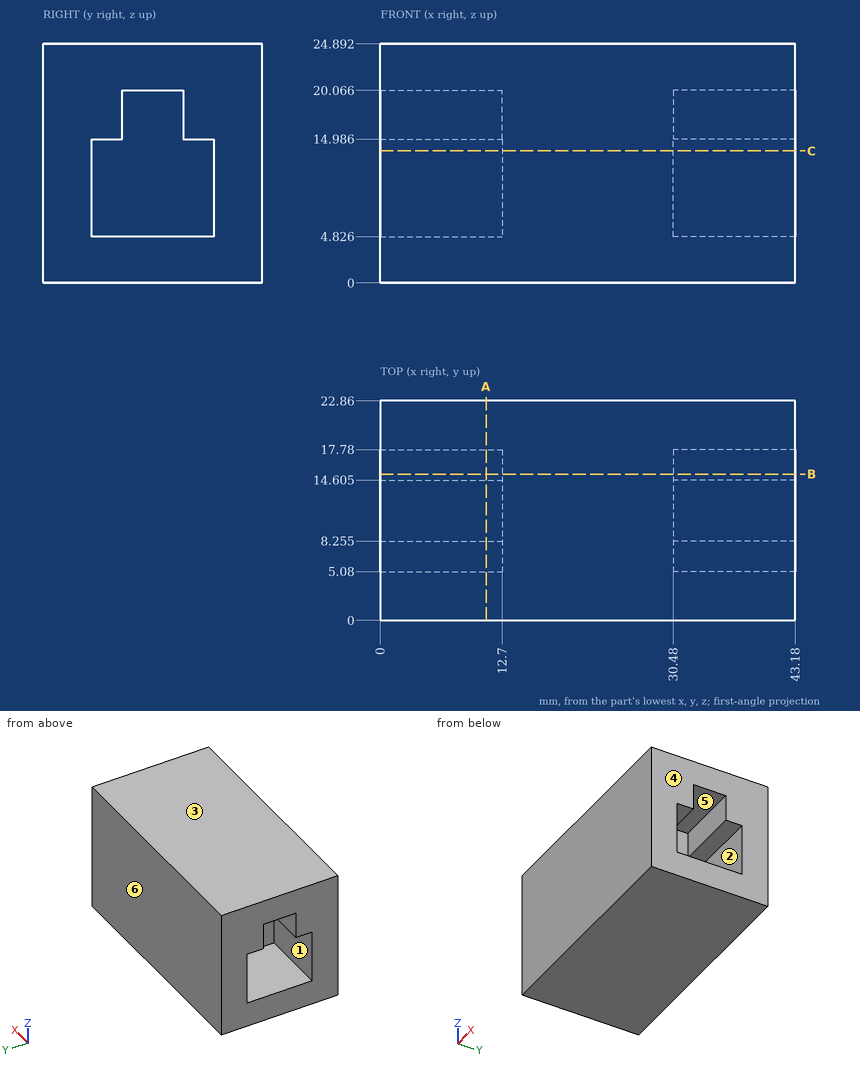
Geometry check sheet. Reference: drawing and pictorial views, mm from the part's lowest x, y, z. A direction names the side the tool comes from. Round coordinates to 2 decimals unless told otherwise and drop trailing zeros. Write each loop counter-clockwise with the first axis right and the second up, starting at its lowest first coordinate (ties: lowest second). Pieces come first, ordered by that corner, then holes.
Item 1: Go/stop test with a flat-tipped pin: pin 1 Ø6.5 at (y, z) = (10.5, 11.5) entering from +X. Record where the tip stops, or that it passes through.
Determined:
pin 1: stops at x = 30.48
Item 2: Material ranges on line 1 along Z through (x, y) = (36, 14); line 2 along Z through (x, y) = (2, 17.5); line 3 along Y through (x, z) = (6.5, 18.5) (3 decimals), recorded low to high.
Determined:
line 1: z = 0 to 4.83, 20.07 to 24.89
line 2: z = 0 to 4.83, 14.99 to 24.89
line 3: y = 0 to 8.255, 14.605 to 22.86
Item 3: Section check B-B (y = 15.25). Record the boundary of the cut face in (x, z), plus the area to 3 significant figures.
Determined:
outline: (0, 0) - (43.18, 0) - (43.18, 4.83) - (30.48, 4.83) - (30.48, 14.99) - (43.18, 14.99) - (43.18, 24.89) - (0, 24.89) - (0, 14.99) - (12.7, 14.99) - (12.7, 4.83) - (0, 4.83) - close
area: 817 mm2
Item 4: Section check C-C (z = 13.75). Record the boundary of the cut face in (x, y).
Determined:
outline: (0, 0) - (43.18, 0) - (43.18, 5.08) - (30.48, 5.08) - (30.48, 17.78) - (43.18, 17.78) - (43.18, 22.86) - (0, 22.86) - (0, 17.78) - (12.7, 17.78) - (12.7, 5.08) - (0, 5.08) - close
Item 5: Mould release check, pull along Y, two halves, no side actions. Record for the marked faces 4, 5 and 6: +Y half, -Y half, draft (parallel to the pull), parting line (faces both ways), or undercut.
Determined:
face 4: draft
face 5: undercut
face 6: +Y half
Item 6: Section check A-A (x = 11). Record the boundary of the cut face in (y, z) (3 decimals).
Determined:
outline: (0, 0) - (22.86, 0) - (22.86, 24.892) - (0, 24.892) - close; hole (5.08, 4.826) - (17.78, 4.826) - (17.78, 14.986) - (14.605, 14.986) - (14.605, 20.066) - (8.255, 20.066) - (8.255, 14.986) - (5.08, 14.986) - close
Item 7: Access from +Z, -Z, +X, -X, +Y, -Y to the whole of each face (thin tool, end or side, straight path). Record for the marked faces 1, 2 and 3.
Determined:
face 1: -X
face 2: +X
face 3: +Z, +X, -X, +Y, -Y
